Geometry: final body of the model. Coordinates: model frame, mm. Face numbers are marked on the shaded views. A direction names the side the tool comes from. Round coordinates to 2 decimals unless told otherwise and drop trailing zeros. Loops run counter-clockwise (first coordinate to the right, second up) from the corner with the lowest first, then second, coordinate; pieces in that order, holes last. Notation, with made-up numbers: M -37,12.5 L -14,12.5 A7 ccw -14,23.5 Z; hole C 74,-6 d3. An arc over 180 degrees is marked long. Answer as a JSON object with one key per item and string values.
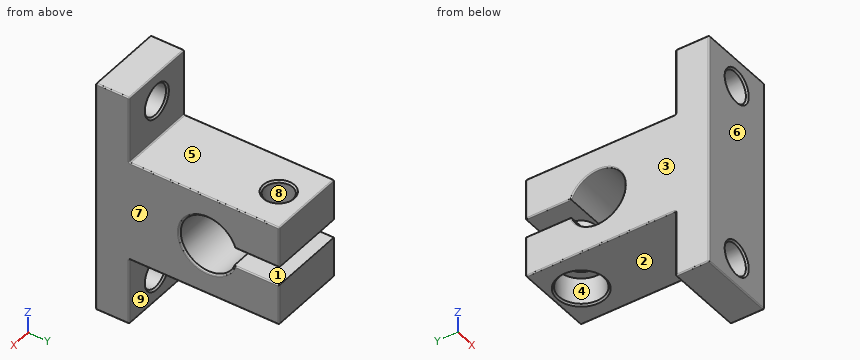
```python
from build123d import *

# Parameters (mm, degrees)
BOSS_EXTRUDE1_DEPTH = 7
SKETCH2_R           = 2.75
CUT_EXTRUDE1_DEPTH  = 7
SKETCH3_R           = 2.5
CUT_EXTRUDE2_DEPTH  = 31
SKETCH4_R           = 4
CUT_EXTRUDE3_DEPTH  = 5
CHAMFER_1_SIZE      = 0.3
FILLET_1_R          = 0.2


with BuildPart() as part:
    # Sketch1 → Boss-Extrude1 (new body, symmetric)
    with BuildSketch(Plane(origin=(0, 0, 0), x_dir=(0, 0, -1), z_dir=(1, 0, 0))):
        with BuildLine():
            Line((-21, 0), (21, 0))
            Line((21, 0), (21, 6))
            Line((21, 6), (9, 6))
            Line((9, 6), (9, 32.8))
            Line((9, 32.8), (1.666666667, 32.8))
            Line((1.666666667, 32.8), (1.666666667, 24.714045208))
            ThreePointArc((1.666666667, 24.714045208), (0, 15), (-1.666666667, 24.714045208))
            Line((-1.666666667, 24.714045208), (-1.666666667, 32.8))
            Line((-1.666666667, 32.8), (-9, 32.8))
            Line((-9, 32.8), (-9, 6))
            Line((-9, 6), (-21, 6))
            Line((-21, 6), (-21, 0))
        make_face()
    extrude(amount=BOSS_EXTRUDE1_DEPTH, both=True)

    # Sketch2 → Cut-Extrude1 (cut, through all)
    with BuildSketch(Plane(origin=(0, 6, 0), x_dir=(1, 0, 0), z_dir=(0, 1, 0))):
        with Locations(Location((0, 16, 0), (0, 0, 270))):  # turned: the seam where the file's is
            Circle(SKETCH2_R)
        with Locations(Location((0, -16, 0), (0, 0, 270))):  # turned: the seam where the file's is
            Circle(SKETCH2_R)
    extrude(amount=-CUT_EXTRUDE1_DEPTH, mode=Mode.SUBTRACT)

    # Sketch3 → Cut-Extrude2 (cut, through all)
    with BuildSketch(Plane(origin=(0, 0, -9), x_dir=(-1, 0, 0), z_dir=(0, 0, -1))):
        with Locations(Location((0, 27.8, 0), (0, 0, 90))):  # turned: the seam where the file's is
            Circle(SKETCH3_R)
    extrude(amount=-CUT_EXTRUDE2_DEPTH, mode=Mode.SUBTRACT)

    # Sketch4 → Cut-Extrude3 (cut)
    with BuildSketch(Plane(origin=(0, 0, -9), x_dir=(-1, 0, 0), z_dir=(0, 0, -1))):
        with Locations((0, 27.8)):
            Circle(SKETCH4_R)
    extrude(amount=-CUT_EXTRUDE3_DEPTH, mode=Mode.SUBTRACT)

    # Фаска1
    chamfer_1_edges = [part.edges().sort_by_distance(p)[0] for p in [
        (7, 15, 0),
        (0, 0, -18.75),
        (0, 6, -18.75),
        (0, 0, 13.25),
        (0, 6, 13.25),
        (0, 25.3, 9),
        (4, 27.8, -9),
    ]]
    chamfer(chamfer_1_edges, length=CHAMFER_1_SIZE)

    # Скругление1
    fillet_1_edges = [part.edges().sort_by_distance(p)[0] for p in [
        (-7, 0, 0),
        (-7, 3, -21),
        (-7, 6, -15),
        (-7, 19.4, -9),
        (-7, 32.8, -5.333333333),
        (-7, 28.757022604, -1.666666667),
        (-7, 15, 0),
        (-7, 28.757022604, 1.666666667),
        (-7, 32.8, 5.333333333),
        (-7, 19.4, 9),
        (-7, 6, 15),
        (-7, 3, 21),
        (7, 32.8, -5.333333333),
        (7, 19.4, -9),
        (7, 6, -15),
        (7, 3, -21),
        (7, 0, 0),
        (7, 3, 21),
        (7, 6, 15),
        (7, 19.4, 9),
        (7, 32.8, 5.333333333),
        (7, 28.915562672, 1.666666667),
        (7, 14.7, 0),
        (7, 28.915562672, -1.666666667),
        (0, 0, 21),
        (0, 6, 21),
        (0, 6, 9),
        (0, 32.8, 9),
        (0, 0, -21),
        (0, 32.8, -9),
        (0, 6, -9),
        (0, 6, -21),
    ]]
    fillet(fillet_1_edges, radius=FILLET_1_R)


solid = part.part
```
1) Cut plane A-A on z = -16. Return the cut outline in (x, y), and give its area (3 significant figures).
Geometry results:
{"outline": "M -7,0.2 A0.2 ccw -6.8,0 L -3.05,0 L -2.75,0.3 L -2.75,5.7 L -3.05,6 L -6.8,6 A0.2 ccw -7,5.8 Z; M 2.75,0.3 L 3.05,0 L 6.8,0 A0.2 ccw 7,0.2 L 7,5.8 A0.2 ccw 6.8,6 L 3.05,6 L 2.75,5.7 Z", "area": "50.8 mm2"}
2) Cut plane C-C on z = 0. Return the cut outline in (x, y).
Geometry results:
{"outline": "M -7,0.2 A0.2 ccw -6.8,0 L 6.8,0 A0.2 ccw 7,0.2 L 7,14.62 A0.2 ccw 6.94,14.76 L 6.7,15 L -6.8,15 A0.2 ccw -7,14.8 Z"}
3) Cut plane B-B on y = 2. Return the cut outline in (x, z), and give its area (3 significant figures).
Geometry results:
{"outline": "M -7,-20.8 A0.2 ccw -6.8,-21 L 6.8,-21 A0.2 ccw 7,-20.8 L 7,20.8 A0.2 ccw 6.8,21 L -6.8,21 A0.2 ccw -7,20.8 Z; hole C 0,-16 d5.5; hole C 0,16 d5.5", "area": "540 mm2"}
4) Cut plane D-D on y = 11.5. Return the cut outline in (x, z).
Geometry results:
{"outline": "M -7,-8.8 A0.2 ccw -6.8,-9 L 6.8,-9 A0.2 ccw 7,-8.8 L 7,8.8 A0.2 ccw 6.8,9 L -6.8,9 A0.2 ccw -7,8.8 Z"}
5) First-contact query: pin 1 (5 mm diameter, centred on x = 0, z = 16, fed in from -Y); pin 2 (6 mm diameter, centred on x = 2, z = -16, fed in from +Y); pin 3 (6 mm diameter, centred on x = -0.5, y = 20.5, fed in from -Z); pin 4 (2.5 mm diameter, centred on x = 0.5, y = 26.5, fed in from -Z). Flat tips, straight axial feed; report the tip coordinate or a pass-through.
Geometry results:
{"pin 1": "through", "pin 2": "y = 6", "pin 3": "z = -9", "pin 4": "z = -4"}
6) Pull-direction query (Y, two-part tool) for the marked faces 6, 7, 8 and 9; classes: +Y half, -Y half, draft (parallel to the pull), parting line (faces both ways), or undercut.
Geometry results:
{"face 6": "-Y half", "face 7": "draft", "face 8": "undercut", "face 9": "+Y half"}
7) Line query: probe 1 along X at (y, z) = (3.2, -16); probe 2 along Z at (x, y) = (-1.75, 25.5); probe 3 along Z at (x, y) = (-1, 20). Output: solid intervals per line, ascending.
Geometry results:
{"probe 1": "-7 to -2.75, 2.75 to 7", "probe 2": "-4 to -1.67, 1.67 to 9", "probe 3": "-9 to -5, 5 to 9"}
8) Set-up query: the marked faces 1, 2, 3, 4 and 5. Return all of +Z, -Z, +X, -X, +Y, -Y with unobstructed straight access to the full face (end or side cutting, diameter ignored); none if empty.
Geometry results:
{"face 1": "+X, -X, +Y", "face 2": "-Z, +X, -X, +Y", "face 3": "+Z, -Z, -X, +Y, -Y", "face 4": "-Z", "face 5": "+Z, +X, -X, +Y"}
